Source: three-view drawing plus pictorial views. Frame: mm from the lowest corner of the part. Round coordinates to 2 decimals unless told otherwise and drop trailing zeros. Loops run counter-clockwise (first coordinate to the right, second up) from the corner with the lowest first, then second, coordinate; pieces in that order, holes last. Notation, with made-up numbers: (39, 89) -> (75, 89) arc R3 ccw to (75, 93) -> close; hole circle Ø5 at (68.5, 57.25). An arc over 180 degrees is marked (long way). Put each result on its own line as item: value. Start each with the question number.
1. Cut plane A-A (y = 184.5). Return the cut outline in (x, z), then the cut area to 3 significant figures.
2. Material intervals for L1, parallel to Y at x = 247, z = 11; L2, parallel to Z at x = 297.5, y = 254.5; L3, parallel to X at y = 398, z = 195.5, sorted ascending.
3. Contact query for flat-ended pins moving along their axis: pin 1 (16 mm diameter, centred on x = 169.5, y = 444, fed in from -Z); pin 2 (6 mm diameter, centred on x = 109, z = 6.5, fed in from -Y); pin 3 (22 mm diameter, centred on x = 9, z = 92, fed in from -Y). Output: stop coordinate, or through.
4. Cut plane B-B (x = 110.5). Return the cut outline in (y, z), then the cut area to 3 significant figures.
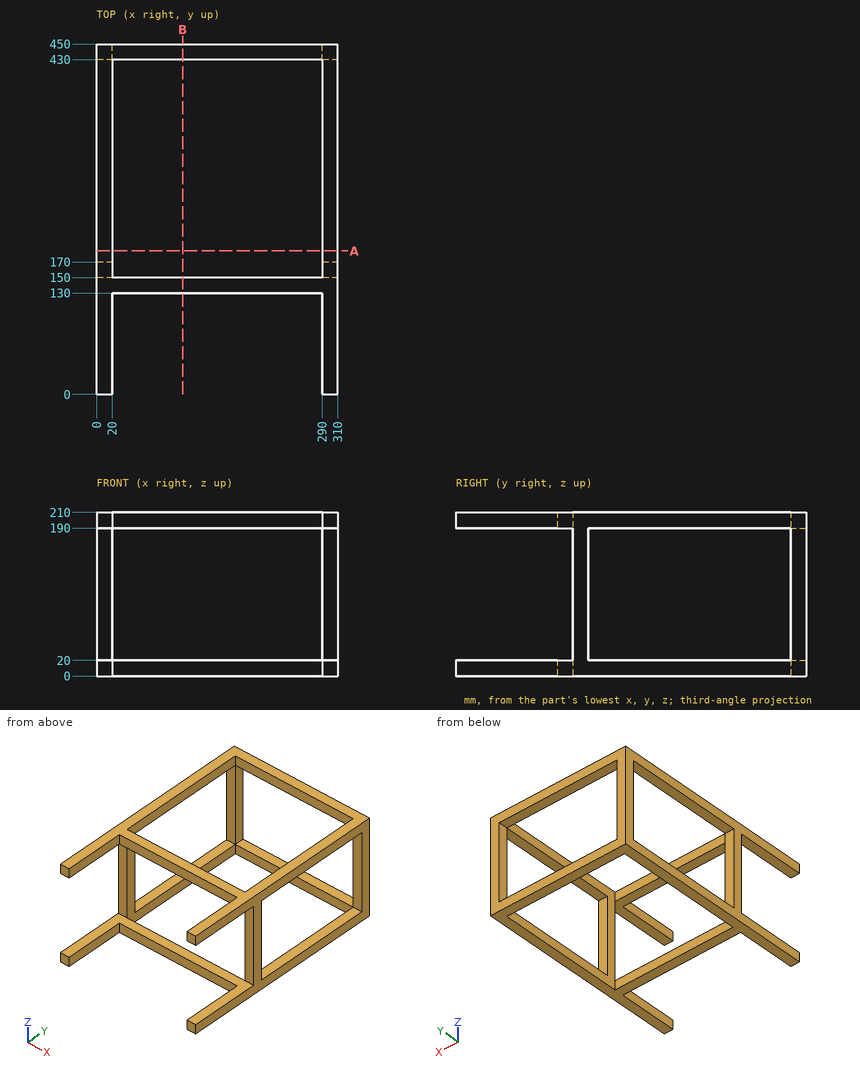
Solution:
1. outline: (0, 0) -> (20, 0) -> (20, 20) -> (0, 20) -> close; (0, 190) -> (20, 190) -> (20, 210) -> (0, 210) -> close; (290, 0) -> (310, 0) -> (310, 20) -> (290, 20) -> close; (290, 190) -> (310, 190) -> (310, 210) -> (290, 210) -> close
1. area: 1,600 mm^2
2. L1: y = 130 to 150, 430 to 450
2. L2: z = 0 to 20, 190 to 210
2. L3: x = 0 to 20, 290 to 310
3. pin 1: stops at z = 0
3. pin 2: stops at y = 130
3. pin 3: stops at y = 150
4. outline: (130, 0) -> (150, 0) -> (150, 20) -> (130, 20) -> close; (130, 190) -> (150, 190) -> (150, 210) -> (130, 210) -> close; (430, 0) -> (450, 0) -> (450, 20) -> (430, 20) -> close; (430, 190) -> (450, 190) -> (450, 210) -> (430, 210) -> close
4. area: 1,600 mm^2
